Could you check a few things on this model? Use its own coordinates, in mm. Give positions to 0.01 mm unless a question says otherwise; leave off trailing zeros. One line per item, written item: value.
```python
from build123d import *

# Parameters (mm, degrees)
BOSS_EXTRUDE1_DEPTH = 460
SKETCH2_W           = 460
SKETCH2_H           = 2.1
SKETCH3_W           = 460
SKETCH3_H           = 2.1


with BuildPart() as part:
    # Sketch1 → Boss-Extrude1 (new body)
    with BuildSketch(Plane.XY):
        with BuildLine():
            Line((-9, -20), (-3, -20))
            Line((-3, -20), (-3, -18))
            Line((-3, -18), (-6, -18))
            Line((-6, -18), (-6, -17.060660172))
            Line((-6, -17.060660172), (-2.939339828, -14))
            Line((-2.939339828, -14), (-0.519615242, -14))
            Line((-0.519615242, -14), (0, -13.7))
            Line((0, -13.7), (0.519615242, -14))
            Line((0.519615242, -14), (2.939339828, -14))
            Line((2.939339828, -14), (6, -17.060660172))
            Line((6, -17.060660172), (6, -18))
            Line((6, -18), (3, -18))
            Line((3, -18), (3, -20))
            Line((3, -20), (9, -20))
            ThreePointArc((9, -20), (9.707106781, -19.707106781), (10, -19))
            Line((10, -19), (10, -13))
            Line((10, -13), (8, -13))
            Line((8, -13), (8, -16))
            Line((8, -16), (7.060660172, -16))
            Line((7.060660172, -16), (4, -12.939339828))
            Line((4, -12.939339828), (4, -10.519615242))
            Line((4, -10.519615242), (3.7, -10))
            Line((3.7, -10), (4, -9.480384758))
            Line((4, -9.480384758), (4, -7.060660172))
            Line((4, -7.060660172), (7.060660172, -4))
            Line((7.060660172, -4), (8, -4))
            Line((8, -4), (8, -7))
            Line((8, -7), (10, -7))
            Line((10, -7), (10, 7))
            Line((10, 7), (8, 7))
            Line((8, 7), (8, 4))
            Line((8, 4), (7.060660172, 4))
            Line((7.060660172, 4), (4, 7.060660172))
            Line((4, 7.060660172), (4, 9.480384758))
            Line((4, 9.480384758), (3.7, 10))
            Line((3.7, 10), (4, 10.519615242))
            Line((4, 10.519615242), (4, 12.939339828))
            Line((4, 12.939339828), (7.060660172, 16))
            Line((7.060660172, 16), (8, 16))
            Line((8, 16), (8, 13))
            Line((8, 13), (10, 13))
            Line((10, 13), (10, 19))
            ThreePointArc((10, 19), (9.707106781, 19.707106781), (9, 20))
            Line((9, 20), (3, 20))
            Line((3, 20), (3, 18))
            Line((3, 18), (6, 18))
            Line((6, 18), (6, 17.060660172))
            Line((6, 17.060660172), (2.939339828, 14))
            Line((2.939339828, 14), (0.519615242, 14))
            Line((0.519615242, 14), (0, 13.7))
            Line((0, 13.7), (-0.519615242, 14))
            Line((-0.519615242, 14), (-2.939339828, 14))
            Line((-2.939339828, 14), (-6, 17.060660172))
            Line((-6, 17.060660172), (-6, 18))
            Line((-6, 18), (-3, 18))
            Line((-3, 18), (-3, 20))
            Line((-3, 20), (-9, 20))
            ThreePointArc((-9, 20), (-9.707106781, 19.707106781), (-10, 19))
            Line((-10, 19), (-10, 13))
            Line((-10, 13), (-8, 13))
            Line((-8, 13), (-8, 16))
            Line((-8, 16), (-7.060660172, 16))
            Line((-7.060660172, 16), (-4, 12.939339828))
            Line((-4, 12.939339828), (-4, 10.519615242))
            Line((-4, 10.519615242), (-3.7, 10))
            Line((-3.7, 10), (-4, 9.480384758))
            Line((-4, 9.480384758), (-4, 7.060660172))
            Line((-4, 7.060660172), (-7.060660172, 4))
            Line((-7.060660172, 4), (-8, 4))
            Line((-8, 4), (-8, 7))
            Line((-8, 7), (-10, 7))
            Line((-10, 7), (-10, -7))
            Line((-10, -7), (-8, -7))
            Line((-8, -7), (-8, -4))
            Line((-8, -4), (-7.060660172, -4))
            Line((-7.060660172, -4), (-4, -7.060660172))
            Line((-4, -7.060660172), (-4, -9.480384758))
            Line((-4, -9.480384758), (-3.7, -10))
            Line((-3.7, -10), (-4, -10.519615242))
            Line((-4, -10.519615242), (-4, -12.939339828))
            Line((-4, -12.939339828), (-7.060660172, -16))
            Line((-7.060660172, -16), (-8, -16))
            Line((-8, -16), (-8, -13))
            Line((-8, -13), (-10, -13))
            Line((-10, -13), (-10, -19))
            ThreePointArc((-10, -19), (-9.707106781, -19.707106781), (-9, -20))
        make_face()
        with BuildLine():
            Line((-7.7, -2), (-7.063603897, -2))
            ThreePointArc((-7.063603897, -2), (-6.948798867, -2.02283614), (-6.851471863, -2.087867966))
            Line((-6.851471863, -2.087867966), (-2.939339828, -6))
            Line((-2.939339828, -6), (2.939339828, -6))
            Line((2.939339828, -6), (6.851471863, -2.087867966))
            ThreePointArc((6.851471863, -2.087867966), (6.948798867, -2.02283614), (7.063603897, -2))
            Line((7.063603897, -2), (7.7, -2))
            ThreePointArc((7.7, -2), (7.912132034, -1.912132034), (8, -1.7))
            Line((8, -1.7), (8, 1.7))
            ThreePointArc((8, 1.7), (7.912132034, 1.912132034), (7.7, 2))
            Line((7.7, 2), (7.063603897, 2))
            ThreePointArc((7.063603897, 2), (6.948798867, 2.02283614), (6.851471863, 2.087867966))
            Line((6.851471863, 2.087867966), (2.939339828, 6))
            Line((2.939339828, 6), (-2.939339828, 6))
            Line((-2.939339828, 6), (-6.851471863, 2.087867966))
            ThreePointArc((-6.851471863, 2.087867966), (-6.948798867, 2.02283614), (-7.063603897, 2))
            Line((-7.063603897, 2), (-7.7, 2))
            ThreePointArc((-7.7, 2), (-7.912132034, 1.912132034), (-8, 1.7))
            Line((-8, 1.7), (-8, -1.7))
            ThreePointArc((-8, -1.7), (-7.912132034, -1.912132034), (-7.7, -2))
        make_face(mode=Mode.SUBTRACT)
    extrude(amount=-BOSS_EXTRUDE1_DEPTH)

    # Sketch2 → Cut-Revolve1 (revolve, cut)
    with BuildSketch(Plane(origin=(0, 0, 0), x_dir=(0, 0, -1), z_dir=(1, 0, 0)), mode=Mode.PRIVATE) as cut_revolve1_sk:
        with Locations((230, 11.05)):
            Rectangle(SKETCH2_W, SKETCH2_H)
    revolve(cut_revolve1_sk.sketch.rotate(Axis((0, 10, -460), (0, 0, 1)), 270), axis=Axis((0, 10, -460), (0, 0, 1)), mode=Mode.SUBTRACT)

    # Sketch3 → Cut-Revolve2 (revolve, cut)
    with BuildSketch(Plane(origin=(0, 0, 0), x_dir=(0, 0, -1), z_dir=(1, 0, 0)), mode=Mode.PRIVATE) as cut_revolve2_sk:
        with Locations((230, -8.95)):
            Rectangle(SKETCH3_W, SKETCH3_H)
    revolve(cut_revolve2_sk.sketch.rotate(Axis((0, -10, -460), (0, 0, 1)), 270), axis=Axis((0, -10, -460), (0, 0, 1)), mode=Mode.SUBTRACT)


solid = part.part
```
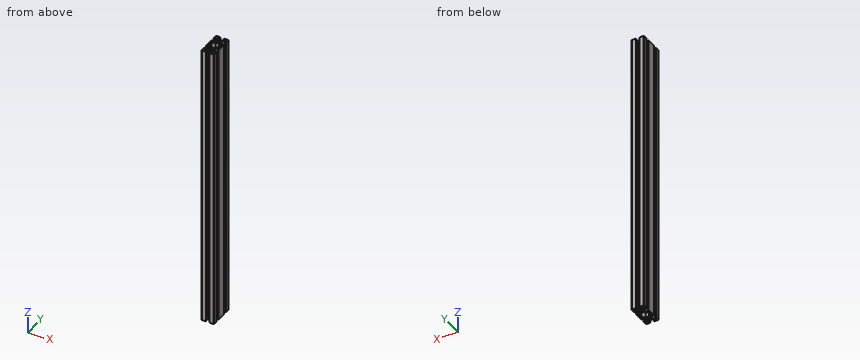
1) Suppose I cut it at A-A, the plane z = -290. State how many separate pieces and enclosed holes the cut face has, then the cut area to 3 significant figures.
Answer below:
separate pieces: 1
enclosed holes: 3
area: 324 mm2
2) If I drill on line 1 along Y through (x, z) = (0, -310.5); line 2 along X through (y, z) = (15, -398); line 3 along Y through (x, z) = (-8.5, -312.5), over which ranges is the centre line in solid material (lowest first)?
Answer below:
line 1: y = -13.7 to -12.1, -7.9 to -6, 6 to 7.9, 12.1 to 13.7
line 2: x = -10 to -8, -6.06 to -3.94, 3.94 to 6.06, 8 to 10
line 3: y = -20 to -13, -7 to 7, 13 to 20
3) For P1, Ø10, axis at x = 1.5, y = 10.5, coming from the -Z side; P2, Ø2, axis at y = -8.5, z = -382.5, coming from the +X side; P3, Ø1.8, axis at x = 0.5, z = -235.5, coming from the +Y side, each with a flat end and sliding along its axis, tell me the tip position at first contact or that it passes through.
Answer below:
P1: stops at z = -460
P2: stops at x = 4
P3: stops at y = 14
